```python
from build123d import *

# Parameters (mm, degrees)
EXTRUSION1_DEPTH = 14
ESQUISSE2_R      = 1.5
EXTRUSION2_DEPTH = 14
ESQUISSE3_R      = 1.5
EXTRUSION3_DEPTH = 14


with BuildPart() as part:
    # Esquisse1 → Extrusion1 (new body)
    with BuildSketch(Plane.XY):
        Polygon((-18.044406835, 3.872316684), (-18.044406835, -11.127683316), (-3.044406835, -11.127683316), (-3.044406835, -9.627683316), (-16.544406835, -9.627683316), (-16.544406835, 3.872316684), align=None)
    extrude(amount=EXTRUSION1_DEPTH)

    # Esquisse2 → Extrusion2 (cut)
    with BuildSketch(Plane(origin=(0, -9.627683316, 0), x_dir=(-1, 0, 0), z_dir=(0, 1, 0))):
        with Locations((8.044406835, 6.5)):
            Circle(ESQUISSE2_R)
    extrude(amount=-EXTRUSION2_DEPTH, mode=Mode.SUBTRACT)

    # Esquisse3 → Extrusion3 (cut)
    with BuildSketch(Plane.ZY.offset(18.044406835)):
        with Locations((6.5, -3.627683316)):
            Circle(ESQUISSE3_R)
    extrude(amount=-EXTRUSION3_DEPTH, mode=Mode.SUBTRACT)


solid = part.part
```
Can you work these out from the model? Positions are in its coordinate system, mm. A direction names the side the tool comes from. Coordinates: 2 decimals unless noted, no trailing zeros. Loops run counter-clockwise (first coordinate to the right, second up) from the corner with the lowest first, then second, coordinate; pieces in that order, holes last. Notation, with made-up numbers: (86.5, -35.75) -> (111.5, -35.75) arc R3 cw to (111.5, -31.75) -> close; hole circle Ø3 at (71.5, -18.75). An arc over 180 degrees is marked (long way). Put each result on its own line as item: value. Start each with the question number.
Q1. I want a section at A-A (z = 6.5). Write out the boundary of the cut face in (x, y).
Q2. For faces 1 (the face through (-10, -9.628, 7)), 2 (the face through (-3.044, -10, 7)), which set-ups out of +Z, -Z, +X, -X, +Y, -Y let a thin tool reach every point of the face, with its end or its side?
Q3. If I drill on line 1 (Y direction, x = -16.85, z = 6.5); line 2 (Y direction, x = -7.75, z = 8.75); line 3 (X direction, y = -8.75, z = 9.25), over which ranges is the centre line in solid material (lowest first)? Write a range as [from, to].
Q4. Thinking about a two-plate mould opening in Z: for faces 3 (the face through (-8.74, -10.37, 5.17)), 4 (the face through (-17.3, -3.6, 5)), 5 (the face through (-17, 3.872, 7)), 6 (the face through (-14, -10, 0)), which applies, pulls with the +Z half, pulls with the -Z half, needs draft (parallel to the pull), parting line crosses it, or undercut?
Q5. I'm going to push flat-ended pins straight in: P1, Ø5, axis at x = -5, z = 3, coming from the +Y side; P2, Ø4, axis at y = 0, z = 6, coming from the +X side; P3, Ø1.8, axis at x = -8.04, z = 6.5, coming from the -Y side; P4, Ø8, axis at x = -14, y = 0, coming from the +Z side. Where does each tip first touch, or does it pass through?
Q6. I want a section at D-D (y = -0.5). Write out the boundary of the cut face in (x, z).
Q7. I want a section at B-B (z = 4.25). Write out the boundary of the cut face in (x, y), plus the area to 4 significant figures.
Q8. I want a section at C-C (x = -3.75). Write out the boundary of the cut face in (y, z).
Taken from the geometry:
1. outline: (-18.04, -11.13) -> (-9.54, -11.13) -> (-9.54, -9.63) -> (-16.54, -9.63) -> (-16.54, -5.13) -> (-18.04, -5.13) -> close; (-18.04, -2.13) -> (-16.54, -2.13) -> (-16.54, 3.87) -> (-18.04, 3.87) -> close; (-6.54, -11.13) -> (-3.04, -11.13) -> (-3.04, -9.63) -> (-6.54, -9.63) -> close
2. face 1: +Z, -Z, +X, +Y
2. face 2: +Z, -Z, +X, +Y, -Y
3. line 1: y = [-11.13, -5.13], [-2.13, 3.87]
3. line 2: y = [-11.13, -9.63]
3. line 3: x = [-18.04, -16.54]
4. face 3: undercut
4. face 4: undercut
4. face 5: needs draft
4. face 6: pulls with the -Z half
5. P1: stops at y = -9.63
5. P2: stops at x = -16.54
5. P3: passes through
5. P4: stops at z = 14
6. outline: (-18.04, 0) -> (-16.54, 0) -> (-16.54, 14) -> (-18.04, 14) -> close
7. outline: (-18.04, -11.13) -> (-3.04, -11.13) -> (-3.04, -9.63) -> (-16.54, -9.63) -> (-16.54, 3.87) -> (-18.04, 3.87) -> close
7. area: 42.75 mm2
8. outline: (-11.13, 0) -> (-9.63, 0) -> (-9.63, 14) -> (-11.13, 14) -> close
